```python
from build123d import *

# Parameters (mm, degrees)
SKETCH1_W              = 240.03
SKETCH1_H              = 360.68
BOSS_EXTRUDE1_DEPTH    = 12.446
M10X1_5_TAPPED_HOLE1_D = 8.5


with BuildPart() as part:
    # Sketch1 → Boss-Extrude1 (new body)
    with BuildSketch(Plane(origin=(0, 0, 0), x_dir=(1, 0, 0), z_dir=(0, 1, 0))):
        Rectangle(SKETCH1_W, SKETCH1_H)
    extrude(amount=BOSS_EXTRUDE1_DEPTH)

    # M10x1.5 Tapped Hole1 (through all)
    with Locations(Plane(origin=(0, 12.446, 0), x_dir=(1, 0, 0), z_dir=(0, 1, 0))):
        with Locations((80.01, 51.435), (80.01, -12.065)):
            m10x1_5_tapped_hole1 = Hole(M10X1_5_TAPPED_HOLE1_D / 2)

    # Mirror1: M10x1.5 Tapped Hole1 across plane
    add(m10x1_5_tapped_hole1.mirror(Plane.ZY), mode=Mode.SUBTRACT)


solid = part.part
```
Geometry: final body of the model. Coordinates: model frame, mm. Coordinates: 2 decimals unless noted, no trailing zeros. Order: outer loops, then holes, each group sorted by start corner. A loop starts at its lowest first (then second) coordinate and runs counter-clockwise, first axis right, second up.
Item 1: Material intervals for line 1 along Z through (x, y) = (80.01, 7.5) (3 decimals), sorted ascending.
Answer:
line 1: z = -180.34 to -55.685, -47.185 to 7.815, 16.315 to 180.34
Item 2: Contact query for flat-ended pins moving along their axis: P1, Ø10, axis at x = -80.01, z = 12.065, coming from the -Y side; P2, Ø7.5, axis at x = 80.01, z = 12.065, coming from the +Y side. Output: stop coordinate, or through.
Answer:
P1: stops at y = 0
P2: passes through
Item 3: Section query A-A (x = 80.01). Output: boundary loops of the cut face in (y, z) (3 decimals).
Answer:
outline: (0, -180.34) - (12.446, -180.34) - (12.446, -55.685) - (0, -55.685) - close; (0, -47.185) - (12.446, -47.185) - (12.446, 7.815) - (0, 7.815) - close; (0, 16.315) - (12.446, 16.315) - (12.446, 180.34) - (0, 180.34) - close
Item 4: Draft query along Z for faces 1 (the face through (-83.383, 6.136, -48.849)), 2 (the face through (-2, 0, -3)), 3 (the face through (-2, 6, 180.34)). Return one class per face: released by +Z, released by -Z, zero draft, split by the parting line, or undercut.
Answer:
face 1: undercut
face 2: zero draft
face 3: released by +Z
